The model under review builds one solid part; all positions refer to its coordinate system, in mm. A direction names the side the tool comes from. Round coordinates to 2 decimals unless told otherwise and drop trailing zeros. Loops run counter-clockwise (first coordinate to the right, second up) from the corner with the lowest first, then second, coordinate; pieces in that order, holes last. Notation, with made-up numbers: M 56.5,28 L 103.5,28 A26 cw 103.5,56 Z; hole C 19.25,-4.75 d8. An arc over 180 degrees is marked long. Answer as a JSON object with one key per item and string values. Group by question number.
Item 1: Insertion check: P1, Ø1, axis at x = 2, y = 3.5, coming from the -Z side; P2, Ø2, axis at x = 2.5, z = -5, coming from the -Y side; P3, Ø6.5, axis at x = 1.5, z = 1, coming from the -Y side. Each pin has a flat end and moves straight along its axis. Give the tip position at first contact, or say it passes through.
Item 2: Tool access review of faces 1 (the face through (2.44, 10.53, 0.54)), 2 (the face through (-2, 0, 9)): name each direction out of +Z, -Z, +X, -X, +Y, -Y from which nothing blocks a thin tool from reaching the whole face with its end or side.
Item 3: Consider section D-D (y = 3). Give the boundary of the cut face in (x, z).
Item 4: Consider section C-C (y = 11.25). Give the boundary of the cut face in (x, z).
Item 5: To check wall thickness, follow line 1 (X direction, y = 9.7, z = 0); line 2 (X direction, y = 2.75, z = 0). State the ranges of each line that lie inside material, in increasing order.
Item 6: Consider section B-B (x = 0). Give the boundary of the cut face in (y, z), and give its area (3 significant figures).
Item 7: Consider section A-A (z = 0). Give the boundary of the cut face in (x, y).
Item 8: The part is to be moulded in two halves that separate along X. For faces 3 (the face through (0, 12.5, 0)), 4 (the face through (9.76, 6.9, 2.17)), 5 (the face through (0, 15, 0)), say which applies: +X half, -X half, draft (parallel to the pull), parting line (faces both ways), or undercut.
```python
from build123d import *

# Parameters (mm, degrees)
FILLET1_R = 1


with BuildPart() as part:
    # Sketch1 → Revolve1 (revolve)
    with BuildSketch(Plane(origin=(0, 0, 0), x_dir=(0, 0, -1), z_dir=(1, 0, 0))):
        Polygon((9, 0), (9, 12.5), (4, 12.5), (4, 8.5), (2.5, 8.5), (2.5, 12.5), (0, 12.5), (0, 15), (10, 15), (10, 0), align=None)
    revolve(axis=Axis((0, 0, 0), (0, 1, 0)))

    # Fillet1
    fillet1_edges = [part.edges().sort_by_distance(p)[0] for p in [
        (0, 15, 10),
    ]]
    fillet(fillet1_edges, radius=FILLET1_R)


solid = part.part
```
Geometry results:
{
 "1": {"P1": "stops at z = -9.89", "P2": "stops at y = 12.5", "P3": "stops at y = 8.5"},
 "2": {"face 1": "-Y", "face 2": "+Z, -Z, +X, -X, -Y"},
 "3": {"outline": "C 0,0 d20; hole C 0,0 d18"},
 "4": {"outline": "C 0,0 d20; C 0,0 d8; hole C 0,0 d18; hole C 0,0 d5"},
 "5": {"line 1": "x = -10 to -9, -4 to -2.5, 2.5 to 4, 9 to 10", "line 2": "x = -10 to -9, 9 to 10"},
 "6": {"outline": "M 0,-10 L 14,-10 A1 ccw 15,-9 L 15,9 A1 ccw 14,10 L 0,10 L 0,9 L 12.5,9 L 12.5,4 L 8.5,4 L 8.5,2.5 L 12.5,2.5 L 12.5,-2.5 L 8.5,-2.5 L 8.5,-4 L 12.5,-4 L 12.5,-9 L 0,-9 Z", "area": "86.6 mm^2"},
 "7": {"outline": "M -10,0 L -9,0 L -9,12.5 L -4,12.5 L -4,8.5 L -2.5,8.5 L -2.5,12.5 L 2.5,12.5 L 2.5,8.5 L 4,8.5 L 4,12.5 L 9,12.5 L 9,0 L 10,0 L 10,14 A1 ccw 9,15 L -9,15 A1 ccw -10,14 Z"},
 "8": {"face 3": "undercut", "face 4": "parting line", "face 5": "draft"}
}
